Source: CAD feature listing. Evaluate the final solid. Frame: model axes, mm. Face numbers are marked on the shaded views. Coordinates: 2 decimals unless noted, no trailing zeros. Order: outer loops, then holes, each group sorted by start corner. A loop starts at its lowest first (then second) coordinate and runs counter-clockwise, first axis right, second up. Notation, with made-up numbers: (-2.5, 60.5) -> (48.5, 60.5) arc R28 ccw to (48.5, 89.5) -> close; hole circle Ø8 at (40.5, -23). An arc over 180 degrees is marked (long way). Write each question's results on one line, items separated by ' | '. Start each with the question number.
from build123d import *

# Parameters (mm, degrees)
F2_T = -1.5
F4_D = 5


with BuildPart() as f1:
    # F0 (on Front) → F1 (revolve)
    with BuildSketch(Plane.XZ):
        Polygon((-22.9846419008, 33.67621309), (-22.9846419008, -36.32378691), (-6.4846419008, -36.32378691), (7.1255733644, 24.1639146534), (8.6255733644, 24.1639146534), (9.515315591, 33.62364854), align=None)
    revolve(axis=Axis((-22.9846419008, 0, -1.32378691), (0, 0, -1)))

    # F2
    f2_openings = [f1.faces().sort_by_distance(p)[0] for p in [
        (-39.234621, 0, 33.649931),
    ]]
    offset(amount=F2_T, openings=f2_openings, kind=Kind.INTERSECTION)

    # F4 (through all)
    with Locations(Plane(origin=(0, 0, -36.32378691), x_dir=(1, 0, 0), z_dir=(0, 0, -1))):
        with Locations((-22.9846419008, 0)):
            Hole(F4_D / 2)


solid = f1.part
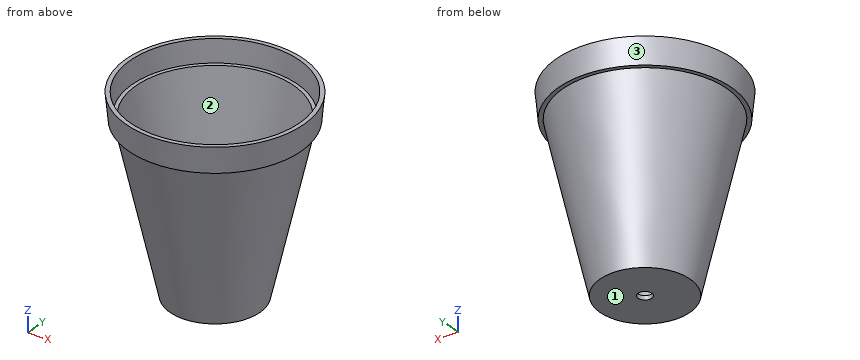
(1) First-contact query: P1, Ø6.5, axis at x = -22.98, y = 0, coming from the +Z side; P2, Ø2, axis at x = 0, z = 0.5, coming from the +Y side; P3, Ø3, axis at x = -17, z = 4.5, coming from the -Y side. Flat tips, straight axial feed; report the tip coordinate or a pass-through.
(2) Line query: L1, parallel to Z at x = -8.5, y = 0.5; L2, parallel to Y at x = -25.5, z = 7; L3, parallel to X at y = 11.5, z = 25. Output: solid intervals per line, ascending.
(3) Section A-A on y = 0. Return the cut outline in (x, z), then the cut area to 3 significant figures.
(4) Section B-B on z = 1. Return the cut outline in (x, y).
(5) Draft query along Y for the marked faces 1, 2 and 3. Return one class per face: released by +Y, released by -Y, zero draft, split by the parting line, or undercut.
(6) Section C-C on z = 10. Return the cut outline in (x, y), then the cut area to 3 significant figures.
Results list:
1) P1: stops at z = -34.82 | P2: stops at y = 11.51 | P3: stops at y = -25.45
2) L1: z = -36.32 to -34.82 | L2: y = -26.13 to -24.58, 24.58 to 26.13 | L3: x = -52.51 to -49.35, 3.38 to 6.54
3) outline: (-55.48, 33.62) -> (-54.59, 24.16) -> (-53.09, 24.16) -> (-39.48, -36.32) -> (-25.48, -36.32) -> (-25.48, -34.82) -> (-38.28, -34.82) -> (-51.89, 25.66) -> (-53.23, 25.66) -> (-53.98, 33.63) -> close; (-20.48, -36.32) -> (-6.48, -36.32) -> (7.13, 24.16) -> (8.63, 24.16) -> (9.52, 33.62) -> (8.01, 33.63) -> (7.26, 25.66) -> (5.93, 25.66) -> (-7.68, -34.82) -> (-20.48, -34.82) -> close | area: 257 mm²
4) outline: circle Ø49.8 at (-22.98, 0); hole circle Ø46.72 at (-22.98, 0)
5) face 1: zero draft | face 2: undercut | face 3: split by the parting line
6) outline: circle Ø53.85 at (-22.98, 0); hole circle Ø50.77 at (-22.98, 0) | area: 253 mm²
